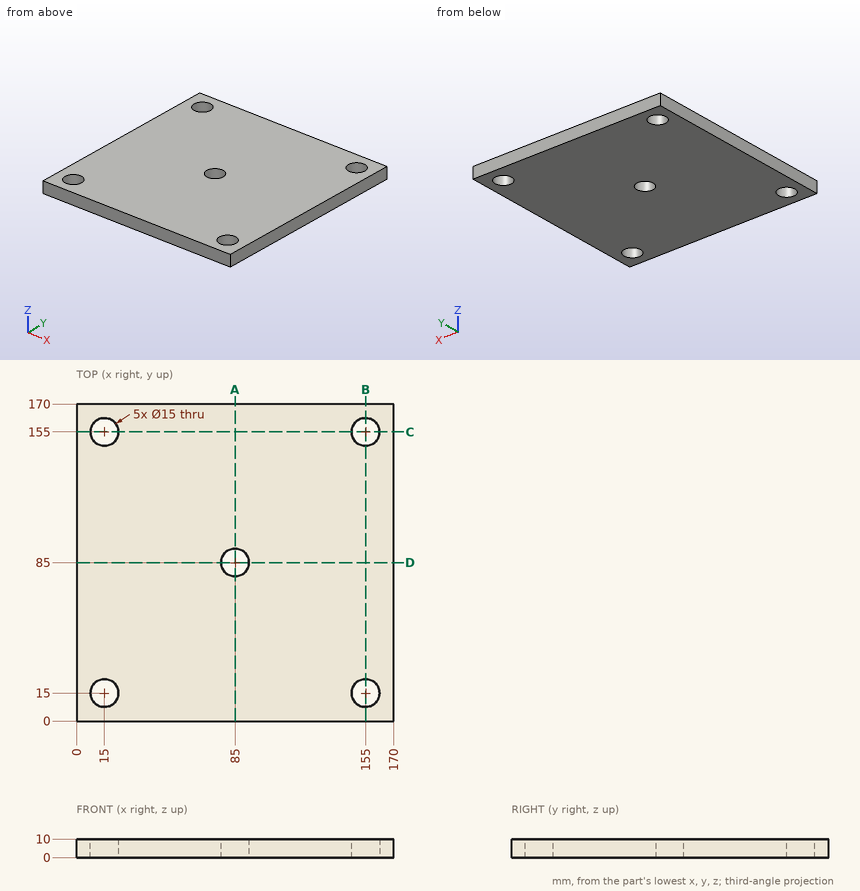
The figure shows three views and two pictorial views of one solid part (mm, origin at its lowest corner). Answer the questions. Coordinates: 2 decimals unless noted, no trailing zeros. Loops run counter-clockwise (first coordinate to the right, second up) from the corner with the lowest first, then second, coordinate; pieces in that order, holes last. Notation, with made-up numbers: (57, 66) -> (97, 66) arc R32 cw to (97, 104) -> close; hole circle Ø5 at (44.25, -2). An arc over 180 degrees is marked (long way). Use one line per item in the form item = value. Start each with the question number.
Item 1: The part is cut by section A-A on x = 85. Determine the outline of the cut face in (y, z).
Item 2: The part is cut by section B-B on x = 155. Determine the outline of the cut face in (y, z), then the cut area to 3 significant figures.
Item 3: Flat-ended cylindrical pins translate along their axes: pin 1 Ø6 at (x, z) = (123, 4) entering from -Y; pin 2 Ø9 at (x, y) = (15, 155) entering from +Z. Find the tip coordinate at first contact, or state that the pin passes through.
Item 4: Consider L1, parallel to X at y = 15, z = 6.25; L2, parallel to X at y = 18, z = 5.25. Determine where each line is inside the solid, lowest interval first. Write a range as [from, to].
Answer key:
q1.outline = (0, 0) -> (77.5, 0) -> (77.5, 10) -> (0, 10) -> close; (92.5, 0) -> (170, 0) -> (170, 10) -> (92.5, 10) -> close
q2.outline = (0, 0) -> (7.5, 0) -> (7.5, 10) -> (0, 10) -> close; (22.5, 0) -> (147.5, 0) -> (147.5, 10) -> (22.5, 10) -> close; (162.5, 0) -> (170, 0) -> (170, 10) -> (162.5, 10) -> close
q2.area = 1,400 mm2
q3.pin_1 = 0
q3.pin_2 = through
q4.L1 = [0, 7.5], [22.5, 147.5], [162.5, 170]
q4.L2 = [0, 8.13], [21.87, 148.13], [161.87, 170]
